Here's the drawing with two shaded views (mm, measured from the low corner). I have some questions. Coordinates: 2 decimals unless noted, no trailing zeros. Write each loop counter-clockwise with the first axis right and the second up, starting at its lowest first coordinate (ties: lowest second). Pieces come first, ordered by that corner, then holes. Notation, with made-up numbers: (-16, -8.75) - (-7, -8.75) arc R17 cw to (-7, 24.25) - close; hole circle Ø6 at (7, -12.75). An arc over 180 degrees is marked (long way). Answer in a Markdown table with one row per item. Add a question column.
Item 1: If I drill on probe 1 along Y at (x, z) = (7.5, 4.5); probe 2 along X at (y, z) = (3.75, 4) (1 decimal); probe 3 along Y at (x, z) = (11.25, 2) (1 decimal), over which ranges is the centre line in solid material (lowest first)? Write a range as from..to.
Item 2: We'd pull the mould along Y, two halves only. Please class the marked faces 1, 2, 3 and 4: +Y half, -Y half, draft (parallel to the pull), parting line (faces both ways), or undercut.
Item 3: I'm going to push flat-ended pins straight in: pin 1 (2.5 mm diameter, centred on x = 7.5, y = 9, fed in from -Z); pin 2 (3 mm diameter, centred on y = 10.5, z = 8, fed in from +X); pin 3 (3 mm diameter, centred on x = 10, z = 3.5, fed in from +Y). Where does each tip first touch, or does it pass through?
Item 4: Imagine slicing it at C-C (x = 7.5). Please give me the cut outline in (y, z).
Item 5: Imagine slicing it at A-A (y = 9). Please give me the cut outline in (x, z), plus the area to 3 significant figures.
Item 6: Imagine slicing it at D-D (y = 3). Please give me the cut outline in (x, z).
Item 7: Imagine slicing it at B-B (z = 8.5). Please give me the cut outline in (x, y).
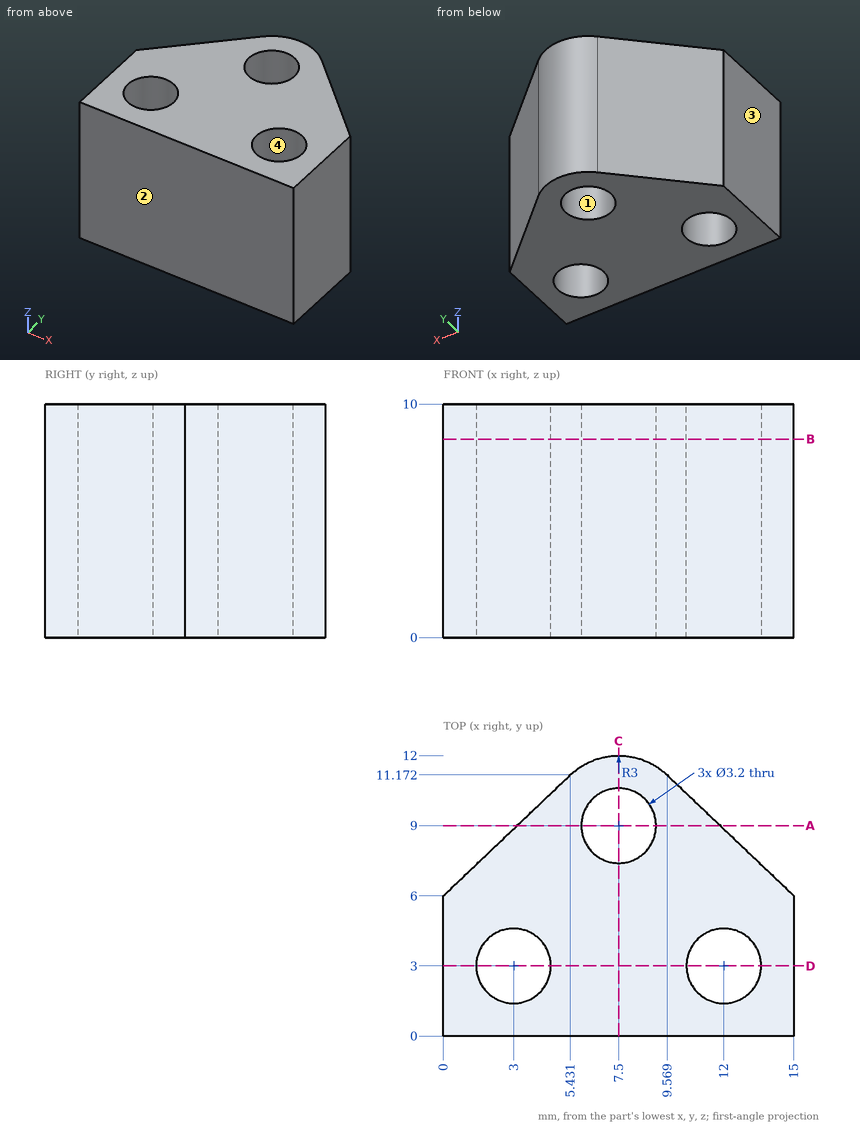
Here are the results:
| question | item | result |
|---|---|---|
| 1 | probe 1 | y = 0..7.4, 10.6..12 |
| 1 | probe 2 | x = 0..1.6, 4.4..10.6, 13.4..15 |
| 1 | probe 3 | y = 0..1.6, 4.4..9.6 |
| 2 | face 1 | undercut |
| 2 | face 2 | -Y half |
| 2 | face 3 | draft |
| 2 | face 4 | undercut |
| 3 | pin 1 | passes through |
| 3 | pin 2 | stops at x = 11.85 |
| 3 | pin 3 | stops at y = 11.83 |
| 4 | outline | (0, 0) - (7.4, 0) - (7.4, 10) - (0, 10) - close; (10.6, 0) - (12, 0) - (12, 10) - (10.6, 10) - close |
| 5 | outline | (3.15, 0) - (5.9, 0) - (5.9, 10) - (3.15, 10) - close; (9.1, 0) - (11.85, 0) - (11.85, 10) - (9.1, 10) - close |
| 5 | area | 55.0 mm2 |
| 6 | outline | (0, 0) - (1.4, 0) - (1.4, 10) - (0, 10) - close; (4.6, 0) - (10.4, 0) - (10.4, 10) - (4.6, 10) - close; (13.6, 0) - (15, 0) - (15, 10) - (13.6, 10) - close |
| 7 | outline | (0, 0) - (15, 0) - (15, 6) - (9.57, 11.17) arc R3 ccw to (5.43, 11.17) - (0, 6) - close; hole circle Ø3.2 at (3, 3); hole circle Ø3.2 at (7.5, 9); hole circle Ø3.2 at (12, 3) |
